The listing builds one solid part. Answer for the finished solid, in the listing's coordinates (mm). Face numbers are marked on the shaded views. A direction names the side the tool comes from. Give positions to 0.01 mm unless a question says otherwise; leave off trailing zeros. Order: outer loops, then holes, each group sorted by start corner. A loop starts at its lowest first (then second) coordinate and runs counter-clockwise, first axis right, second up. Notation, with made-up numbers: (48.5, 48.5) - (72.5, 48.5) arc R13 ccw to (72.5, 59.5) - close; hole circle Ø11 at (88.25, 49). An arc over 180 degrees is marked (long way). Write each question's results on one line, items separated by ' | '. Start each with the question number.
1. Flat-ended cylindrical pins translate along their axes: pin 1 (6 mm diameter, centred on x = -86.5, y = 11, fed in from +Z); pin 2 (9.5 mm diameter, centred on x = 180, y = 18, fed in from +Z); pin 3 (4.5 mm diameter, centred on y = 4, z = 39, fed in from -X). Find the tip coordinate at first contact, or state that the pin passes through.
2. Determine the mould class of the marked faces 1, 2 and 3 for opening direction Z: released by +Z, released by -Z, zero draft, split by the parting line, or undercut.
3. Section B-B (x = 49.5) is taken. Give the vertices of the cut face in (y, z).
4. Find the intervals of material crossed by L1, parallel to Z at x = 27, y = 12; L2, parallel to Y at x = -12, z = -1.15; L3, parallel to Z at x = -157, y = 30, in increasing order.
5. Which of the six approach directions +Z, -Z, +X, -X, +Y, -Y give full straight-line access (tool end or side, diameter ignored) to the marked faces 4 and 5?
6. Section A-A (z = 135.5) is taken. Give the vertices of the cut face in (x, y).
7. Section C-C (z = 16) is taken. Give the vertices of the cut face in (x, y).
from build123d import *

# Parameters (mm, degrees)
SKETCH_1_W               = 378
SKETCH_1_H               = 35
EXTRUDE_1_DEPTH          = 2.5
SKETCH_3_W               = 4
SKETCH_3_H               = 35
EXTRUDE_2_DEPTH          = 35
SKETCH_4_R               = 2.55
CUT_EXTRUDE_3_DEPTH      = 382.464611727
HOLE_WIZARD_M4_6_D       = 3.3
SKETCH_6_W               = 30
SKETCH_6_H               = 15
EXTRUDE_3_DEPTH          = 200
EXTRUDE_4_REACH          = 385.676
SKETCH_15_W              = 20
SKETCH_15_H              = 15
EXTRUDE_5_REACH          = 428.74
SKETCH_17_W              = 4
SKETCH_17_H              = 35
SKETCH_18_W              = 4
SKETCH_18_H              = 35
EXTRUDE_6_DEPTH          = 185
CUT_EXTRUDE_4_DEPTH      = 410.325359586
CUT_EXTRUDE_4_DEPTH_BACK = 410.325359586
FILLET_1_R               = 100
FILLET_2_R               = 10
RIB_6_REACH              = 398.424
SKETCH_20_WALL_W         = 836.856433298
SKETCH_20_WALL_H         = 15


with BuildPart() as part:
    # 草图1 → 凸台-拉伸1 (new, symmetric)
    with BuildSketch(Plane.XY):
        with Locations((0, 17.5)):
            Rectangle(SKETCH_1_W, SKETCH_1_H)
    extrude(amount=EXTRUDE_1_DEPTH, both=True)

    # 草图3 → 凸台-拉伸2 (add)
    with BuildSketch(Plane(origin=(0, 0, -2.5), x_dir=(-1, 0, 0), z_dir=(0, 0, -1))):
        with Locations((-187, 17.5)):
            Rectangle(SKETCH_3_W, SKETCH_3_H)
        with Locations((187, 17.5)):
            Rectangle(SKETCH_3_W, SKETCH_3_H)
    extrude(amount=EXTRUDE_2_DEPTH)

    # 草图4 → 切除-拉伸3 (cut, through all)
    with BuildSketch(Plane(origin=(189, 0, 0), x_dir=(0, 0, -1), z_dir=(1, 0, 0))):
        with Locations((17.5, 17.5)):
            Circle(SKETCH_4_R)
    extrude(amount=-CUT_EXTRUDE_3_DEPTH, mode=Mode.SUBTRACT)

    # M4 螺纹孔的螺纹孔钻头6 (through all)
    with Locations(Plane.XY.offset(2.5)):
        with Locations((12, 27), (-12, 9), (-12, 27), (12, 9)):
            Hole(HOLE_WIZARD_M4_6_D / 2)

    # 草图6 → 凸台-拉伸3 (add)
    with BuildSketch(Plane.XY.offset(2.5)):
        with Locations((-150, 7.5)):
            Rectangle(SKETCH_6_W, SKETCH_6_H)
        with Locations((150, 7.5)):
            Rectangle(SKETCH_6_W, SKETCH_6_H)
    extrude(amount=EXTRUDE_3_DEPTH)

    # 草图15 → 凸台-拉伸4 (add, up to next)
    with BuildSketch(Plane(origin=(-135, 0, 0), x_dir=(0, 0, -1), z_dir=(1, 0, 0)), mode=Mode.PRIVATE) as extrude_4_sk1:
        with Locations((-86.382417222, 7.5)):
            Rectangle(SKETCH_15_W, SKETCH_15_H)
    extrude_4_tool1 = extrude(extrude_4_sk1.sketch, amount=EXTRUDE_4_REACH, mode=Mode.PRIVATE) - part.part
    add(extrude_4_tool1.solids().sort_by_distance((-135, 7.5, 86.382417))[0])

    # 草图17 → 凸台-拉伸5 (add, up to next)
    with BuildSketch(Plane.ZY.offset(-185), mode=Mode.PRIVATE) as extrude_5_sk1:
        with Locations((-35.5, 17.5)):
            Rectangle(SKETCH_17_W, SKETCH_17_H)
    extrude_5_tool1 = extrude(extrude_5_sk1.sketch, amount=EXTRUDE_5_REACH, mode=Mode.PRIVATE) - part.part
    add(extrude_5_tool1.solids().sort_by_distance((185, 17.5, -35.5))[0])

    # 草图18 → 凸台-拉伸6 (add)
    with BuildSketch(Plane(origin=(-185, 0, 0), x_dir=(0, 0, -1), z_dir=(1, 0, 0))):
        with Locations((35.5, 17.5)):
            Rectangle(SKETCH_18_W, SKETCH_18_H)
    extrude(amount=EXTRUDE_6_DEPTH)

    # 草图19 → 切除-拉伸4 (cut, two sides: drawn at the far end of the back side and taken through both)
    with BuildSketch(Plane.ZY.offset(165).offset(-CUT_EXTRUDE_4_DEPTH_BACK)):
        Polygon((-247.587382518, 262.210386508), (180.593567073, 15), (202.5, 2.352315052), (630.680949591, -244.858071456), (1125.101722607, 611.503827726), (246.833390498, 1118.57228569), align=None)
    extrude(amount=CUT_EXTRUDE_4_DEPTH + CUT_EXTRUDE_4_DEPTH_BACK, mode=Mode.SUBTRACT)

    # 圆角1
    # the kernel refuses this fillet: 100 mm, written as the material it takes off along each edge
    with BuildSketch(Plane(origin=(-212.264366854, 2.352315052, 202.5), x_dir=(0, -1, 0), z_dir=(1, 0, 0)), Plane(origin=(87.735633146, 2.352315052, 202.5), x_dir=(0, -1, 0), z_dir=(1, 0, 0))) as fillet_1_piece_1:
        with BuildLine():
            CenterArc((77.149667008, 66.372856956), FILLET_1_R, 210, 11.584858497)
            Line((-9.452873371, 16.372856956), (-11.184924178, 15.372856956))
            Line((-11.184924178, 15.372856956), (-1.732050808, -1))
            Line((-1.732050808, -1), (0, -2))
            ThreePointArc((0, -2), (1.176157526, -2), (0.856368013, -1.327457139))
            Line((0.856368013, -1.327457139), (2.352315052, 0))
        make_face()
    extrude(amount=124.528733709, mode=Mode.SUBTRACT)

    # 圆角2
    fillet_2_edges = [part.edges().sort_by_distance(p)[0] for p in [
        (150, 15, 180.593567073),
        (-150, 15, 180.593567073),
    ]]
    fillet(fillet_2_edges, radius=FILLET_2_R)

    # 草图20 wall → 筋6 (add, up to next)
    with BuildSketch(Plane(origin=(150, 25, 20.970604306), x_dir=(0, -0.476102376571, 0.879389860655), z_dir=(0, -0.879389860655, -0.476102376571)), mode=Mode.PRIVATE) as rib_6_sk1:
        Rectangle(SKETCH_20_WALL_W, SKETCH_20_WALL_H)
    rib_6_tool1 = extrude(rib_6_sk1.sketch, amount=RIB_6_REACH, mode=Mode.PRIVATE) - part.part
    rib_6 = rib_6_tool1.solids().sort_by_distance((150, 25, 20.970604306))[0]
    add(rib_6)

    # 镜向1: 筋6 across plane
    add(rib_6.mirror(Plane(origin=(0, 0, 0), x_dir=(0, 0, 1), z_dir=(1, 0, 0))))


solid = part.part
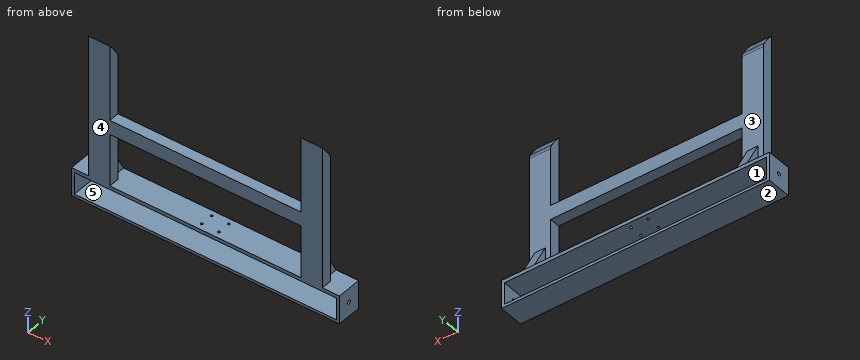
Reported:
1) pin 1: z = 96.38 | pin 2: z = 2.5 | pin 3: x = -165
2) face 1: undercut | face 2: released by -Z | face 3: zero draft
3) outline: (0, -37.5) - (35, -37.5) - (35, -33.5) - (0, -33.5) - close; (0, -2.5) - (35, -2.5) - (35, 2.5) - (0, 2.5) - close; (0, 76.38) - (15, 76.38) - (15, 96.38) - (0, 96.38) - close
4) L1: -37.5 to -33.5, -2.5 to 2.5, 76.38 to 96.38 | L2: 0 to 7.35, 10.65 to 25.35, 28.65 to 35 | L3: -37.5 to -33.5, -2.5 to 11.74
5) face 4: +Z, -Z, +X, -X, -Y | face 5: +Y, -Y
6) outline: (-165, 0) - (-135, 0) - (-135, 15) - (-165, 15) - close; (135, 0) - (165, 0) - (165, 15) - (135, 15) - close
7) outline: (-165, 0) - (-135, 0) - (-135, 15) - (-142.5, 15) - (-142.5, 27.69) - (-157.5, 27.69) - (-157.5, 15) - (-165, 15) - close; (135, 0) - (165, 0) - (165, 15) - (157.5, 15) - (157.5, 27.69) - (142.5, 27.69) - (142.5, 15) - (135, 15) - close
